The listing builds one solid part. Answer for the finished solid, in the listing's coordinates (mm). Face numbers are marked on the shaded views. A direction names the side the tool comes from. Coordinates: 2 decimals unless noted, no trailing zeros. Order: outer loops, then holes, each group sorted by start corner. A loop starts at its lowest first (then second) coordinate and runs counter-clockwise, first axis right, second up. Notation, with made-up numbers: (37, 22.5) -> (50, 22.5) arc R21 cw to (50, 47.5) -> close; hole circle Ø8 at (21, 56.5). An arc over 180 degrees is marked (long way). Put each result on its own line as item: value. Start each with the question number.
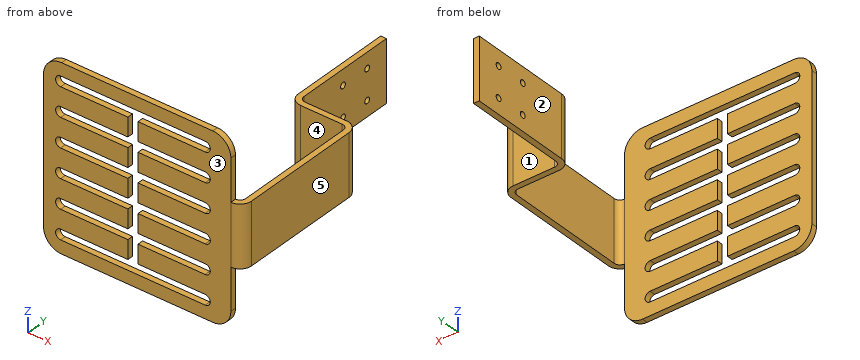
```python
from build123d import *

# Parameters (mm, degrees)
BRIDA_BASE1_DEPTH           = 75
CORTAR_EXTRUIR1_START       = -9.525
CORTAR_EXTRUIR1_OUTLINE_W   = 49.6
CORTAR_EXTRUIR1_OUTLINE_H   = 121
CORTAR_EXTRUIR1_DEPTH       = 9.525
CORTAR_EXTRUIR1_START_2     = -53.5025
CORTAR_EXTRUIR1_2_OUTLINE_W = 49.6
CORTAR_EXTRUIR1_2_OUTLINE_H = 94.7625
CORTAR_EXTRUIR1_2_DEPTH     = 43.9775
CORTAR_EXTRUIR2_DEPTH       = 10
CORTAR_EXTRUIR3_DEPTH       = 10
REDONDEO1_R                 = 15


# Read off the part's stored shape, not the designer's step: Cortar-Extruir1
# Sheet-metal steps are written as plain solids
with BuildPart() as part:
    # Croquis1 → Brida base1 (new, symmetric)
    with BuildSketch(Plane.XY):
        with BuildLine():
            Line((33.76, 105), (33.76, 19.7625))
            ThreePointArc((33.76, 19.7625), (35.154903955, 16.394903955), (38.5225, 15))
            Line((38.5225, 15), (72.975, 15))
            ThreePointArc((72.975, 15), (79.710192091, 12.210192091), (82.5, 5.475))
            Line((82.5, 5.475), (82.5, -95.475))
            ThreePointArc((82.5, -95.475), (79.710192091, -102.210192091), (72.975, -105))
            Line((72.975, -105), (-82.5, -105))
            Line((-82.5, -105), (-82.5, -100.2375))
            Line((-82.5, -100.2375), (72.975, -100.2375))
            ThreePointArc((72.975, -100.2375), (76.342596045, -98.842596045), (77.7375, -95.475))
            Line((77.7375, -95.475), (77.7375, 5.475))
            ThreePointArc((77.7375, 5.475), (76.342596045, 8.842596045), (72.975, 10.2375))
            Line((72.975, 10.2375), (38.5225, 10.2375))
            ThreePointArc((38.5225, 10.2375), (31.787307909, 13.027307909), (28.9975, 19.7625))
            Line((28.9975, 19.7625), (28.9975, 105))
            Line((28.9975, 105), (33.76, 105))
        make_face()
    extrude(amount=BRIDA_BASE1_DEPTH, both=True)

    # Cortar-Extruir1 outline → Cortar-Extruir1 (cut)
    with BuildSketch(Plane(origin=(82.5, 0, 0), x_dir=(0, 0, -1), z_dir=(1, 0, 0)).offset(CORTAR_EXTRUIR1_START)):
        with Locations((50.2, -45.5)):
            Rectangle(CORTAR_EXTRUIR1_OUTLINE_W, CORTAR_EXTRUIR1_OUTLINE_H)
        with Locations((-50.2, -45.5)):
            Rectangle(CORTAR_EXTRUIR1_OUTLINE_W, CORTAR_EXTRUIR1_OUTLINE_H)
    extrude(amount=CORTAR_EXTRUIR1_DEPTH, mode=Mode.SUBTRACT)

    # Cortar-Extruir1 2 outline → Cortar-Extruir1 2 (cut)
    with BuildSketch(Plane(origin=(82.5, 0, 0), x_dir=(0, 0, -1), z_dir=(1, 0, 0)).offset(CORTAR_EXTRUIR1_START_2)):
        with Locations((50.2, 57.61875)):
            Rectangle(CORTAR_EXTRUIR1_2_OUTLINE_W, CORTAR_EXTRUIR1_2_OUTLINE_H)
        with Locations((-50.2, 57.61875)):
            Rectangle(CORTAR_EXTRUIR1_2_OUTLINE_W, CORTAR_EXTRUIR1_2_OUTLINE_H)
    extrude(amount=CORTAR_EXTRUIR1_2_DEPTH, mode=Mode.SUBTRACT)

    # Croquis7 → Cortar-Extruir2 (cut)
    with BuildSketch(Plane(origin=(33.76, 0, 0), x_dir=(0, 0, -1), z_dir=(1, 0, 0))):
        with BuildLine():
            ThreePointArc((-15, 84.9995), (-12.5, 82.4995), (-10, 84.9995))
            ThreePointArc((-10, 84.9995), (-12.5, 87.5005), (-15, 84.9995))
        make_face()
        with BuildLine():
            ThreePointArc((10, 84.9995), (12.5, 82.4995), (15, 84.9995))
            ThreePointArc((15, 84.9995), (12.5, 87.5005), (10, 84.9995))
        make_face()
        with BuildLine():
            ThreePointArc((10, 59.9995), (12.5, 57.4995), (15, 59.9995))
            ThreePointArc((15, 59.9995), (12.5, 62.5005), (10, 59.9995))
        make_face()
        with BuildLine():
            ThreePointArc((-15, 59.9995), (-12.5, 57.4995), (-10, 59.9995))
            ThreePointArc((-10, 59.9995), (-12.5, 62.5005), (-15, 59.9995))
        make_face()
    extrude(amount=-CORTAR_EXTRUIR2_DEPTH, mode=Mode.SUBTRACT)

    # Croquis8 → Cortar-Extruir3 (cut)
    with BuildSketch(Plane.XZ.offset(105)):
        with BuildLine():
            Line((-68.3, -64.2), (51.7, -64.2))
            ThreePointArc((51.7, -64.2), (55.9, -60), (51.7, -55.8))
            Line((51.7, -55.8), (-4.1, -55.8))
            Line((-4.1, -55.8), (-4.1, -40.2))
            Line((-4.1, -40.2), (51.7, -40.2))
            ThreePointArc((51.7, -40.2), (55.9, -36), (51.7, -31.8))
            Line((51.7, -31.8), (-4.1, -31.8))
            Line((-4.1, -31.8), (-4.1, -16.2))
            Line((-4.1, -16.2), (51.7, -16.2))
            ThreePointArc((51.7, -16.2), (55.9, -12), (51.7, -7.8))
            Line((51.7, -7.8), (-4.1, -7.8))
            Line((-4.1, -7.8), (-4.1, 7.8))
            Line((-4.1, 7.8), (51.7, 7.8))
            ThreePointArc((51.7, 7.8), (55.9, 12), (51.7, 16.2))
            Line((51.7, 16.2), (-4.1, 16.2))
            Line((-4.1, 16.2), (-4.1, 31.8))
            Line((-4.1, 31.8), (51.7, 31.8))
            ThreePointArc((51.7, 31.8), (55.9, 36), (51.7, 40.2))
            Line((51.7, 40.2), (-4.1, 40.2))
            Line((-4.1, 40.2), (-4.1, 55.8))
            Line((-4.1, 55.8), (51.7, 55.8))
            ThreePointArc((51.7, 55.8), (55.9, 60), (51.7, 64.2))
            Line((51.7, 64.2), (-68.3, 64.2))
            ThreePointArc((-68.3, 64.2), (-72.5, 60), (-68.3, 55.8))
            Line((-68.3, 55.8), (-12.5, 55.8))
            Line((-12.5, 55.8), (-12.5, 40.2))
            Line((-12.5, 40.2), (-68.3, 40.2))
            ThreePointArc((-68.3, 40.2), (-72.5, 36), (-68.3, 31.8))
            Line((-68.3, 31.8), (-12.5, 31.8))
            Line((-12.5, 31.8), (-12.5, 16.2))
            Line((-12.5, 16.2), (-68.3, 16.2))
            ThreePointArc((-68.3, 16.2), (-72.5, 12), (-68.3, 7.8))
            Line((-68.3, 7.8), (-12.5, 7.8))
            Line((-12.5, 7.8), (-12.5, -7.8))
            Line((-12.5, -7.8), (-68.3, -7.8))
            ThreePointArc((-68.3, -7.8), (-72.5, -12), (-68.3, -16.2))
            Line((-68.3, -16.2), (-12.5, -16.2))
            Line((-12.5, -16.2), (-12.5, -31.8))
            Line((-12.5, -31.8), (-68.3, -31.8))
            ThreePointArc((-68.3, -31.8), (-72.5, -36), (-68.3, -40.2))
            Line((-68.3, -40.2), (-12.5, -40.2))
            Line((-12.5, -40.2), (-12.5, -55.8))
            Line((-12.5, -55.8), (-68.3, -55.8))
            ThreePointArc((-68.3, -55.8), (-72.5, -60), (-68.3, -64.2))
        make_face()
    extrude(amount=-CORTAR_EXTRUIR3_DEPTH, mode=Mode.SUBTRACT)

    # Redondeo1
    redondeo1_edges = [part.edges().sort_by_distance(p)[0] for p in [
        (-82.5, -102.61875, -75),
        (72.975, -102.61875, -75),
        (72.975, -102.61875, 75),
        (-82.5, -102.61875, 75),
    ]]
    fillet(redondeo1_edges, radius=REDONDEO1_R)


solid = part.part
```
(1) The part is cut by section B-B on z = -36. Determine the outline of the cut face in (x, y) (1 decimal).
(2) Find the intervals of material crossed by L1, parallel to Y at x = 5.5, z = 49; L2, parallel to X at y = 75.5, z = -25; L3, parallel to X at y = -86, z = 0, in increasing order.
(3) Each of these flat-tipped pins is pushed along its axis until it touches: P1, Ø4, axis at y = 46, z = 16, coming from the +X side; P2, Ø8, axis at x = -55, z = 16, coming from the -Y side; P3, Ø1.4, axis at y = -102.5, z = 44.5, coming from the +X side (3 decimals); P4, Ø8, axis at x = 27, z = -46.5, coming from the +Y side. Where does it stop, or does it pass through?
(4) A tool of negligible diameter and unlimited length cuts with its end or side. For the marked faces 1, 2, 3, 4 and 5, from which of +Z, -Z, +X, -X, +Y, -Y can it reach the whole face along a straight path? Write none if from no direction.
(5) The part is cut by section A-A on x = 26.5. Determine the outline of the cut face in (y, z).
(6) The part is cut by section C-C on x = 47. Count the separate pieces of the cut face and the enclosed holes in it, plus the area to 3 significant figures.
Worked out:
1. outline: (-82.5, -105) -> (-72.5, -105) -> (-72.5, -100.2) -> (-82.5, -100.2) -> close; (55.9, -105) -> (73, -105) -> (73, -100.2) -> (55.9, -100.2) -> close
2. L1: -105 to -100.24
2. L2: 29 to 33.76
2. L3: 77.74 to 82.5
3. P1: x = 33.76
3. P2: y = -105
3. P3: x = 72.975
3. P4: y = -100.24
4. face 1: +Z, -Z, +X, +Y
4. face 2: +Z, -Z, -X, +Y
4. face 3: +Z, -Z, +X, -X, -Y
4. face 4: +Z, -Z, -X
4. face 5: +Z, -Z, +X, +Y, -Y
5. outline: (-105, -75) -> (-100.24, -75) -> (-100.24, -64.2) -> (-105, -64.2) -> close; (-105, -55.8) -> (-100.24, -55.8) -> (-100.24, -40.2) -> (-105, -40.2) -> close; (-105, -31.8) -> (-100.24, -31.8) -> (-100.24, -16.2) -> (-105, -16.2) -> close; (-105, -7.8) -> (-100.24, -7.8) -> (-100.24, 7.8) -> (-105, 7.8) -> close; (-105, 16.2) -> (-100.24, 16.2) -> (-100.24, 31.8) -> (-105, 31.8) -> close; (-105, 40.2) -> (-100.24, 40.2) -> (-100.24, 55.8) -> (-105, 55.8) -> close; (-105, 64.2) -> (-100.24, 64.2) -> (-100.24, 75) -> (-105, 75) -> close
6. separate pieces: 8
6. enclosed holes: 0
6. area: 716 mm2
